Part model, mm, in its own coordinate system. Round coordinates to 2 decimals unless told otherwise and drop trailing zeros. Loops run counter-clockwise (first coordinate to the right, second up) from the corner with the lowest first, then second, coordinate; pieces in that order, holes last. Notation, with made-up numbers: (74, -16.5) -> (97, -16.5) arc R16 cw to (97, -3.5) -> close; hole circle Ø1 at (30, 4.5). An arc over 180 degrees is marked (long way). Answer as a JSON object with one key per item and string values. Group by question number.
from build123d import *

# Parameters (mm, degrees)
SKETCH1_R           = 2.5
BOSS_EXTRUDE1_DEPTH = 2.5
CIRPATTERN1_COUNT   = 2


with BuildPart() as part:
    # Sketch1 → Boss-Extrude1 (new, symmetric)
    with BuildSketch(Plane(origin=(0, 0, 0), x_dir=(1, 0, 0), z_dir=(0, 1, 0))):
        with BuildLine():
            ThreePointArc((0, 5), (5, 0), (0, -5))
            Line((0, -5), (0, -17.5))
            add(Edge.make_bspline(
                [(0, -17.5), (26.944118738, -17.53258197), (52.619662803, -29.065950844), (80, -22.5)],
                knots=[0, 0, 0, 0, 1, 1, 1, 1], degree=3))
            ThreePointArc((80, -22.5), (217.756302371, -17.591386703), (355.6, -17.5))
            Line((355.6, -17.5), (355.6, -8.75))
            ThreePointArc((355.6, -8.75), (347.367245335, 2.896213541), (335, 10))
            add(Edge.make_bspline(
                [(335, 10), (239.516107029, 20.502209099), (143.75, 22)],
                knots=[0, 0, 0, 0.750368183, 0.750368183, 0.750368183], degree=2))
            Line((143.75, 22), (80, 22))
            ThreePointArc((80, 22), (40.077104301, 18.379256879), (0, 17.5))
            Line((0, 17.5), (0, 5))
        make_face()
        with Locations(Location((7.209644007, -6.929721011, 0), (0, 0, 270))):
            Circle(SKETCH1_R, mode=Mode.SUBTRACT)
        with Locations(Location((7.209644007, 6.929721011, 0), (0, 0, 270))):
            Circle(SKETCH1_R, mode=Mode.SUBTRACT)
    boss_extrude1 = extrude(amount=BOSS_EXTRUDE1_DEPTH, both=True)

    # CirPattern1: Boss-Extrude1 ×2 about axis
    cirpattern1_axis = Axis((0, -2.5, 0), (0, 1, 0))
    for i in range(1, CIRPATTERN1_COUNT):
        add(boss_extrude1.rotate(cirpattern1_axis, i * 360 / CIRPATTERN1_COUNT))


solid = part.part
Item 1: Drill centre lines: line 1 (X direction, y = 1.95, z = -8); line 2 (X direction, y = 0.4, z = 4); line 3 (Z direction, x = 0, y = -0.3). Where is each one in solid material? Low to high.
Item 2: Band-saw the part on B-B, the plane x = -121. List the corners of the cut face in (y, z).
Item 3: Band-saw the part on A-A, the plane y = -1.65. Count the separate pieces of the cut face and the enclosed holes in it, plus the area to 3 significant figures.
Item 4: Drop flat-ended pins along their axis: pin 1 Ø2.5 at (x, y) = (-107.5, 0.5) entering from +Z; pin 2 Ø2 at (y, z) = (1.5, -10) entering from +X; pin 3 Ø8 at (x, z) = (-7.21, 6.93) entering from -Y. Give the stop position or say it passes through.
Entries:
{
 "1": {"line 1": "-355.27 to -9.47, -4.95 to 4.95, 9.47 to 339.94", "line 2": "-346.09 to -3, 3 to 353.13", "line 3": "-17.5 to -5, 5 to 17.5"},
 "2": {"outline": "(-2.5, -20.53) -> (2.5, -20.53) -> (2.5, 22) -> (-2.5, 22) -> close"},
 "3": {"separate pieces": "1", "enclosed holes": "5", "area": "26,100 mm²"},
 "4": {"pin 1": "z = 22", "pin 2": "x = 337.75", "pin 3": "y = -2.5"}
}
